Geometry check sheet. Reference: the model listing, model coordinates, mm. Face numbers are marked on the shaded views. A direction names the side the tool comes from. Coordinates: 2 decimals unless noted, no trailing zeros. Order: outer loops, then holes, each group sorted by start corner. A loop starts at its lowest first (then second) coordinate and runs counter-clockwise, first axis right, second up. Notation, with made-up numbers: (-13, 2) - (-5, 2) arc R27 ccw to (-5, 33) - close; hole circle Ø1 at (62, 17.5). An arc over 180 degrees is marked (long way). Use CSV: the item, a comma, the result in double quotes. Start each with the question number.
1) Draft check along Z on the marked faces 4, 5 and 6. Enter one of: released by +Z, released by -Z, zero draft, split by the parting line, or undercut.
2) Tool access check on the marked faces 1, 2 and 3. Record the directions out of +Z, -Z, +X, -X, +Y, -Y that give a thin tool (end or side, any length) a straight path to the whole face; none if there is none.
3) Sectioned sample at D-D, the plane x = -47.5. Record the cut outline in (y, z).
4) Depth check by flat-ended pin: P1, Ø11, axis at y = -4.5, z = 5, coming from the +X side; P2, Ø2, axis at x = -29.5, z = -2, coming from the +Y side; P3, Ø23, axis at y = 0, z = 0, coming from the -X side; P4, Ø17.5, axis at y = 0, z = 0, coming from the -X side. Enter the tip coordinate at first touch or a pass-through.
5) Thickness scan on probe 1 along Y at (x, z) = (-24.5, 0); probe 2 along Y at (x, z) = (-18, 0); probe 3 along Z at (x, y) = (-8.5, 2.5). Record the ranges inside material, lowest first. Write a range as [from, to].
6) Sectioned sample at C-C, the plane x = -20.5. Record the cut outline in (y, z).
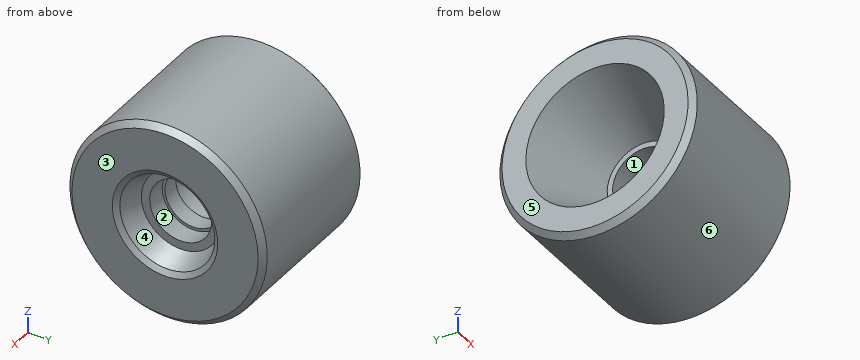
from build123d import *


# Not quite as in the source:
# - a fillet or chamfer that OpenCascade refuses, or shapes differently, is made with other operations: its cross-section is extruded or revolved along the edge and cut away or added


with BuildPart() as f1:
    # F0 (on Front) → F1 (revolve)
    with BuildSketch(Plane.XZ):
        Polygon((-15.7733729929, 11), (-8.7733729929, 11), (-8.7733729929, 13.9589581495), (0, 17.3333312895), (0, 35), (-56, 35), (-56, 24.5486367494), (-28.7733729929, 12.9255643114), (-28.7733729929, 11), (-21.7733729929, 11), (-21.7733729929, 10), (-15.7733729929, 10), align=None)
    revolve(axis=Axis((-19.2243028432, 0, 0), (-1, 0, 0)))

    # F2: chamfer of 2 on 3 edges, made by hand

    # F2_s1 → F2_t2 (revolve, cut)
    with BuildSketch(Plane.XZ):
        Polygon((0, 33), (-2, 35), (0, 35), align=None)
    revolve(axis=Axis((0, 0, 0), (-1, 0, 0)), mode=Mode.SUBTRACT)

    # F2_s3 → F2_t4 (revolve, cut)
    with BuildSketch(Plane.XZ):
        Polygon((-54, 35), (-56, 33), (-56, 35), align=None)
    revolve(axis=Axis((-56, 0, 0), (-1, 0, 0)), mode=Mode.SUBTRACT)

    # F2_s5 → F2_t6 (revolve, cut)
    with BuildSketch(Plane.XZ):
        Polygon((-1.2820420431, 16.840238355), (0, 18.706929645), (0, 17.3333312895), align=None)
    revolve(axis=Axis((0, 0, 0), (-1, 0, 0)), mode=Mode.SUBTRACT)


solid = f1.part
Evaluation:
1,face 4,"undercut"
1,face 5,"zero draft"
1,face 6,"split by the parting line"
2,face 1,"-X"
2,face 2,"+X"
2,face 3,"+Z, -Z, +X, +Y, -Y"
3,outline,"circle Ø70 at (0, 0); hole circle Ø41.84 at (0, 0)"
4,P1,"x = -8.77"
4,P2,"y = 34.99"
4,P3,"x = -28.77"
4,P4,"through"
5,probe 1,"[-35, -11], [11, 35]"
5,probe 2,"[-35, -10], [10, 35]"
5,probe 3,"[-34.91, -13.84], [13.84, 34.91]"
6,outline,"circle Ø70 at (0, 0); hole circle Ø20 at (0, 0)"
